Work out the finished part from the listing and answer in its coordinate system (mm). Give positions to 0.01 mm unless a question says otherwise; leave off trailing zeros. Write each loop counter-clockwise with the first axis right and the second up, starting at its lowest first coordinate (ties: lowest second). Pieces come first, ordered by that corner, then holes.
1) Given pin 1 Ø3 at (x, y) = (24.5, -38) entering from +Z; pin 2 Ø2 at (x, y) = (2.5, -18) entering from +Z; pin 3 Ø4 at (x, z) = (59.5, -2) entering from -Y, each flat-ended and moving along its own axis, determine where each tip first touches the part or whether it passes through.
2) Find section A-A (y = -44.5). Determine the outline of the cut face in (x, z).
3) Determine the mould class of faces 1 (the face through (-2.17, -23.66, -9.76)), 2 (the face through (10, -50, -10)), 3 (the face through (81.965, -1.875, -6.161)), 4 (the face through (47.16, -12.32, -21.1)) for opening direction Z: pulls with the +Z half, pulls with the -Z half, needs draft (parallel to the pull), parting line crosses it, or undercut.
4) Find section C-C (x = 90). Determine the outline of the cut face in (y, z), plus the area to 3 significant figures.
5) Find section B-B (y = -8). Determine the outline of the cut face in (x, z).
6) Straight lines are drawn through the part: probe 1 along Z at (x, y) = (0, -37.5); probe 2 along Z at (x, y) = (90, -15); probe 3 along X at (y, z) = (-23, 2). For each, find the intervals that lie inside material, in ascending order.
7) Find section D-D (z = -1.5). Count the separate pieces of the cut face and the enclosed holes in it, plus the area to 3 significant figures.
```python
from build123d import *

# Parameters (mm, degrees)
F0_R        = 10
F1_DEPTH    = 25
F2_DEPTH    = 50
F3_T4_ANGLE = 203.6133668192
F3_T6_ANGLE = 179.9906971182


# Not quite as in the source:
# - a fillet or chamfer that OpenCascade refuses, or shapes differently, is made with other operations: its cross-section is extruded or revolved along the edge and cut away or added


with BuildPart() as f1:
    # F0 (on Front) → F1 (new body)
    with BuildSketch(Plane.XZ):
        with BuildLine():
            Line((4.1054428346, 24.6606029758), (0, 25))
            ThreePointArc((0, 25), (-25, 0), (0, -25))
            Line((0, -25), (4.1054428346, -24.6606029758))
            ThreePointArc((4.1054428346, -24.6606029758), (19.0740146648, -16.1611251022), (25, 0))
            ThreePointArc((25, 0), (19.0740146648, 16.1611251022), (4.1054428346, 24.6606029758))
        make_face()
        Circle(F0_R, mode=Mode.SUBTRACT)
        with BuildLine():
            ThreePointArc((4.1054428346, 24.6606029758), (2.0597239626, 24.9150062653), (0, 25))
            Line((0, 25), (4.1054428346, 24.6606029758))
        make_face()
        with BuildLine():
            Line((4.1054428346, -24.6606029758), (0, -25))
            ThreePointArc((0, -25), (2.0597239626, -24.9150062653), (4.1054428346, -24.6606029758))
        make_face()
        with BuildLine():
            Line((91.4418067738, 17.4405043857), (4.1054428346, 24.6606029758))
            ThreePointArc((4.1054428346, 24.6606029758), (19.0740146648, 16.1611251022), (25, 0))
            ThreePointArc((25, 0), (19.0740146648, -16.1611251022), (4.1054428346, -24.6606029758))
            Line((4.1054428346, -24.6606029758), (91.4418067738, -17.4405043857))
            ThreePointArc((91.4418067738, -17.4405043857), (72.5, 0), (91.4418067738, 17.4405043857))
        make_face()
        with BuildLine():
            ThreePointArc((107.5, 0), (102.8740362463, 11.8536572723), (91.4418067738, 17.4405043857))
            ThreePointArc((91.4418067738, 17.4405043857), (72.5, 0), (91.4418067738, -17.4405043857))
            ThreePointArc((91.4418067738, -17.4405043857), (102.8740362463, -11.8536572723), (107.5, 0))
        make_face()
        with Locations((90, 0)):
            Circle(F0_R, mode=Mode.SUBTRACT)
    extrude(amount=F1_DEPTH)

    # F0 (on Front) → F2 (join)
    with BuildSketch(Plane.XZ):
        with BuildLine():
            Line((4.1054428346, 24.6606029758), (0, 25))
            ThreePointArc((0, 25), (-25, 0), (0, -25))
            Line((0, -25), (4.1054428346, -24.6606029758))
            ThreePointArc((4.1054428346, -24.6606029758), (19.0740146648, -16.1611251022), (25, 0))
            ThreePointArc((25, 0), (19.0740146648, 16.1611251022), (4.1054428346, 24.6606029758))
        make_face()
        Circle(F0_R, mode=Mode.SUBTRACT)
    extrude(amount=F2_DEPTH)

    # F3: chamfer of 2 on 5 edges, made by hand

    # F3_s1 → F3_t2 (revolve, cut)
    with BuildSketch(Plane.XY):
        Polygon((12, -50), (10, -48), (10, -50), align=None)
    revolve(axis=Axis((0, -50, 0), (0, -1, 0)), mode=Mode.SUBTRACT)

    # F3_s3 → F3_t4 (revolve, cut)
    with BuildSketch(Plane(origin=(0, 0, 0), x_dir=(0, 1, 0), z_dir=(0.9788435281, 0, -0.2046102329))):
        Polygon((-48, 25), (-50, 23), (-50, 25), align=None)
    revolve(axis=Axis((0, -50, 0), (0, -1, 0)), revolution_arc=F3_T4_ANGLE, mode=Mode.SUBTRACT)

    # F3_s5 → F3_t6 (revolve, cut)
    with BuildSketch(Plane(origin=(0, 0, 0), x_dir=(0, 1, 0), z_dir=(-0.9999999967, 0, 8.1183e-05))):
        Polygon((-48, -25), (-50, -23), (-50, -25), align=None)
    revolve(axis=Axis((0, -50, 0), (0, 1, 0)), revolution_arc=F3_T6_ANGLE, mode=Mode.SUBTRACT)

    # F3_s7 → F3_t8 (revolve, cut)
    with BuildSketch(Plane.XY):
        Polygon((100, -2), (102, 0), (100, 0), align=None)
    revolve(axis=Axis((90, 0, 0), (0, -1, 0)), mode=Mode.SUBTRACT)

    # F3_s9 → F3_t10 (revolve, cut)
    with BuildSketch(Plane.XY):
        Polygon((102, -25), (100, -23), (100, -25), align=None)
    revolve(axis=Axis((90, -25, 0), (0, -1, 0)), mode=Mode.SUBTRACT)


solid = f1.part
```
Results:
1. pin 1: stops at z = 9.8
1. pin 2: stops at z = 24.95
1. pin 3: stops at y = -25
2. outline: (0, -25) - (4.11, -24.66) arc R25 ccw to (4.11, 24.66) - (0, 25) arc R25 ccw to start; hole circle Ø20 at (0, 0)
3. face 1: undercut
3. face 2: needs draft
3. face 3: undercut
3. face 4: pulls with the -Z half
4. outline: (-25, -17.56) - (0, -17.56) - (0, -12) - (-2, -10) - (-23, -10) - (-25, -12) - close; (-25, 12) - (-23, 10) - (-2, 10) - (0, 12) - (0, 17.56) - (-25, 17.56) - close
4. area: 370 mm2
5. outline: (4.11, -24.66) - (91.44, -17.44) arc R17.5 ccw to (91.44, 17.44) - (4.11, 24.66) arc R25 ccw (long way) to start; hole circle Ø20 at (0, 0); hole circle Ø20 at (90, 0)
6. probe 1: z = -25 to -10, 10 to 25
6. probe 2: z = -17.56 to -10, 10 to 17.56
6. probe 3: x = -24.92 to -9.8, 9.8 to 80.2, 99.8 to 107.39
7. separate pieces: 3
7. enclosed holes: 0
7. area: 3,060 mm2
